Model file for the job. Use its own axes, mm. Face numbers are marked on the shaded views. A direction names the side the tool comes from. Round coordinates to 2 decimals unless told otherwise and drop trailing zeros. Loops run counter-clockwise (first coordinate to the right, second up) from the corner with the lowest first, then second, coordinate; pieces in that order, holes last. Notation, with made-up numbers: (-9, -2) - (6, -2) arc R34 ccw to (6, 32) - close; hole circle Ø1 at (51.5, 23). An arc over 180 degrees is marked (long way). Use one line per item in the form item = value.
from build123d import *

# Parameters (mm, degrees)
PAD_DEPTH     = 10
SKETCH001_R   = 15
PAD001_DEPTH  = 30
SKETCH002_R   = 10
PAD002_DEPTH  = 20
SKETCH003_R   = 7
SKETCH003_R_2 = 11
POCKET_DEPTH  = 30.001
PAD003_DEPTH  = 5


with BuildPart() as part:
    # Sketch → Pad (new body)
    with BuildSketch(Plane.XY):
        with BuildLine():
            ThreePointArc((-13.297973, 14.4138), (-24.146408, -1e-06), (-13.297971, -14.4138))
            Line((30.687086, -27.081719), (-13.297971, -14.4138))
            ThreePointArc((30.687086, -27.081719), (66.669258, 1.3e-05), (30.687062, 27.081712))
            Line((-13.297973, 14.4138), (30.687062, 27.081712))
        make_face()
    extrude(amount=PAD_DEPTH)

    # Sketch001 → Pad001 (join)
    with BuildSketch(Plane.XY):
        with Locations((38.486743, 0)):
            Circle(SKETCH001_R)
    extrude(amount=PAD001_DEPTH)

    # Sketch002 → Pad002 (join)
    with BuildSketch(Plane.XY):
        with Locations((-9.146726, 0)):
            Circle(SKETCH002_R)
    extrude(amount=PAD002_DEPTH)

    # Sketch003 → Pocket (cut, through all)
    with BuildSketch(Plane.XY):
        with Locations((-9.146726, 0)):
            Circle(SKETCH003_R)
        with Locations((38.486743, 0)):
            Circle(SKETCH003_R_2)
    extrude(amount=POCKET_DEPTH, mode=Mode.SUBTRACT)

    # Sketch004 (on DatumPlane) → Pad003 (join, symmetric)
    with BuildSketch(Plane(origin=(6.731097, 0, 0.333333), x_dir=(-1, 0, 0), z_dir=(0, 1, 0))):
        Polygon((-16.755646, 29.666667), (5.877823, 19.666667), (7.877823, 19.666667), (7.877823, 9.666667), (-18.755646, 9.666667), (-18.755646, 29.666667), align=None)
    extrude(amount=PAD003_DEPTH, both=True)


solid = part.part
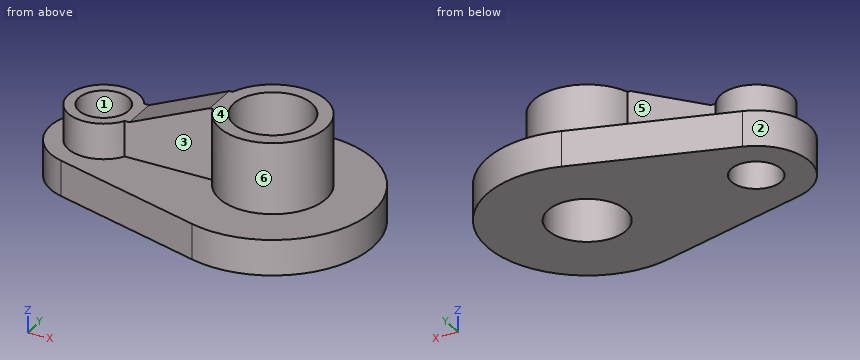
1. Pull direction Y, two halves, no side cores. Call the marked faces 1, 2 and 3: +Y half, -Y half, draft (parallel to the pull), parting line (faces both ways), or undercut.
Geometry check:
face_1 = undercut
face_2 = parting line
face_3 = -Y half
2. Wall check: probe 1 along X at (y, z) = (0, 11); probe 2 along X at (y, z) = (0, 8.5); probe 3 along Z at (x, y) = (29.5, -18.5). Give the ranges that are in metal, low to high.
Geometry check:
probe_1 = -19.15 to -16.15, -2.15 to 27.49, 49.49 to 53.49
probe_2 = -24.15 to -16.15, -2.15 to 27.49, 49.49 to 66.67
probe_3 = 0 to 10
3. Flat gauge pins, fed straight in: pin 1 (2 mm diameter, centred on y = -21.5, z = 3.5, fed in from +X); pin 2 (8 mm diameter, centred on x = 10.5, y = 7.5, fed in from +Z); pin 3 (4 mm diameter, centred on x = 8, y = 7.5, fed in from +Z); pin 4 (8.5 mm diameter, centred on x = -9.15, y = 0, fed in from +Z). Where does each tip first touch, or does it go through?
Geometry check:
pin_1 = 57.83
pin_2 = 25.64
pin_3 = 10
pin_4 = through
4. Cut at C-C, the plane z = 8.5. Give the cut face in (x, y).
Geometry check:
outline = (-13.3, -14.41) - (30.69, -27.08) arc R28.18 ccw (long way) to (30.69, 27.08) - (-13.3, 14.41) arc R15 ccw to start; hole circle Ø14 at (-9.15, 0); hole circle Ø22 at (38.49, 0)
5. Tool access for the marked faces 4, 5 and 6: list every direction of +Z, -Z, +X, -X, +Y, -Y with a clear straight run to the whole face (end or side of a thin tool).
Geometry check:
face_4 = +Z, +X, -X, +Y, -Y
face_5 = +Z, +Y
face_6 = +Z
6. Cut at B-B, the plane y = 9. Give the cut face in (x, z).
Geometry check:
outline = (-21.15, 0) - (32.16, 0) - (32.16, 30) - (26.49, 30) - (26.49, 10) - (-4.79, 10) - (-4.79, 20) - (-13.51, 20) - (-13.51, 10) - (-21.15, 10) - close; (44.81, 0) - (65.19, 0) - (65.19, 10) - (50.49, 10) - (50.49, 30) - (44.81, 30) - close
7. Cut at D-D, the plane x = 38. Give the cut face in (y, z).
Geometry check:
outline = (-28.18, 0) - (-10.99, 0) - (-10.99, 30) - (-14.99, 30) - (-14.99, 10) - (-28.18, 10) - close; (10.99, 0) - (28.18, 0) - (28.18, 10) - (14.99, 10) - (14.99, 30) - (10.99, 30) - close
8. Cut at A-A, the plane y = 0. Give the cut face in (x, z).
Geometry check:
outline = (-24.15, 0) - (-16.15, 0) - (-16.15, 20) - (-19.15, 20) - (-19.15, 10) - (-24.15, 10) - close; (-2.15, 0) - (27.49, 0) - (27.49, 30) - (23.49, 30) - (0.85, 20) - (-2.15, 20) - close; (49.49, 0) - (66.67, 0) - (66.67, 10) - (53.49, 10) - (53.49, 30) - (49.49, 30) - close
